Model file for the job. Use its own axes, mm. Face numbers are marked on the shaded views. A direction names the side the tool comes from. Give positions to 0.01 mm unless a question says otherwise; leave off trailing zeros. Order: outer loops, then holes, each group sorted by start corner. A loop starts at its lowest first (then second) coordinate and runs counter-clockwise, first axis right, second up. Notation, with made-up numbers: (87.5, 25.25) - (94.5, 25.25) arc R8 ccw to (94.5, 36.25) - close; hole circle Ø9 at (14, 69). An arc over 180 degrees is marked (long way). Use CSV: the item, a comma, the result in double quotes. Start each with the question number.
(1) Band-saw the part on B-B, the plane x = 1. Give the cut face in (y, z).
(2) Band-saw the part on A-A, the plane z = 4. Give the cut face in (x, y).
(3) Probe L1, parallel to X at y = -6, z = 5.25; L2, parallel to X at y = -10, z = 2; L3, parallel to Y at x = 3, z = 5.75. List the from-to ranges inside material, lowest first.
(4) Band-saw the part on D-D, the plane y = -6. Give the cut face in (x, z), then the cut area to 3 significant figures.
(5) Band-saw the part on C-C, the plane z = 0.5. Give the cut face in (x, y).
(6) Drop flat-ended pins along their axis: pin 1 Ø4.5 at (x, y) = (3.5, -4) entering from +Z; pin 2 Ø2 at (x, z) = (29, 5) entering from -Y. Give the stop position or say it passes through.
(7) Tool access for the marked faces 4, 5 and 6: list every direction of +Z, -Z, +X, -X, +Y, -Y with a clear straight run to the whole face (end or side of a thin tool).
(8) Pull direction X, two halves, no side cores. Call the marked faces 1, 2 and 3: +X half, -X half, draft (parallel to the pull), parting line (faces both ways), or undercut.
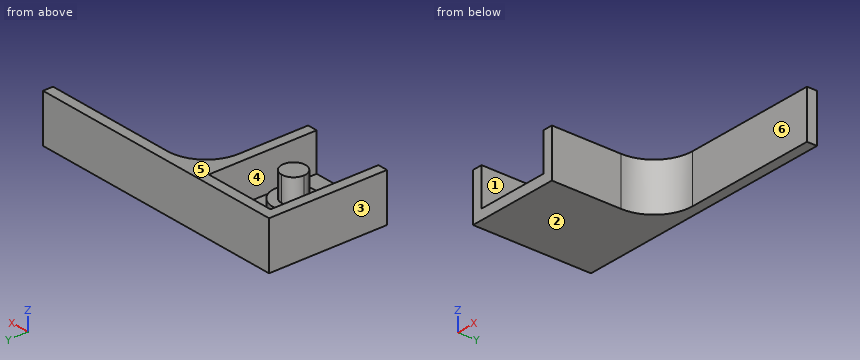
from build123d import *

# Parameters (mm, degrees)
F1_DEPTH = 6.2
F0_W     = 1.3
F0_H     = 14
F2_DEPTH = 3
F3_DEPTH = 1.3
F4_R     = 5


with BuildPart() as f1:
    # F0 (on Top) → F1 (new body)
    with BuildSketch(Plane.XY):
        with BuildLine():
            ThreePointArc((6.25, -7), (5.7960155108, -5.9039844892), (4.7, -5.45))
            Line((4.7, -5.45), (4.7, -7))
            Line((4.7, -7), (3.15, -7))
            ThreePointArc((3.15, -7), (4.7, -8.55), (6.25, -7))
        make_face()
        with BuildLine():
            Line((4.7, -7), (4.7, -5.45))
            ThreePointArc((4.7, -5.45), (3.6039844892, -5.9039844892), (3.15, -7))
            Line((3.15, -7), (4.7, -7))
        make_face()
    extrude(amount=F1_DEPTH)

    # F0 (on Top) → F2 (join)
    with BuildSketch(Plane.XY):
        with BuildLine():
            ThreePointArc((7.4, -7), (6.6091883092, -5.0908116908), (4.7, -4.3))
            Line((4.7, -4.3), (4.7, -5.45))
            ThreePointArc((4.7, -5.45), (5.7960155108, -5.9039844892), (6.25, -7))
            ThreePointArc((6.25, -7), (4.7, -8.55), (3.15, -7))
            Line((3.15, -7), (2, -7))
            ThreePointArc((2, -7), (4.7, -9.7), (7.4, -7))
        make_face()
        with BuildLine():
            Line((4.7, -5.45), (4.7, -4.3))
            ThreePointArc((4.7, -4.3), (2.7908116908, -5.0908116908), (2, -7))
            Line((2, -7), (3.15, -7))
            ThreePointArc((3.15, -7), (3.6039844892, -5.9039844892), (4.7, -5.45))
        make_face()
    extrude(amount=F2_DEPTH)



with BuildPart() as f1b:
    # F0 (on Top) → F1, piece 2 (new body)
    with BuildSketch(Plane.XY):
        Polygon((0, -7), (0, 0), (-1.3, 0), (-1.3, -14), (0, -14), align=None)
        with Locations((10.05, -7)):
            Rectangle(F0_W, F0_H)
        Polygon((-1.3, 0), (0, 0), (4.7, 0), (9.4, 0), (10.7, 0), (33.1, 0), (33.1, 1.3), (-1.3, 1.3), align=None)
    extrude(amount=F1_DEPTH)


with BuildPart() as f1_1:
    add(f1.part)

    add(f1b.part)  # F3 merges F1b
    # F0 (on Top) → F3 (join)
    with BuildSketch(Plane.XY):
        with BuildLine():
            Line((9.4, 0), (4.7, 0))
            Line((4.7, 0), (4.7, -4.3))
            ThreePointArc((4.7, -4.3), (6.6091883092, -5.0908116908), (7.4, -7))
            ThreePointArc((7.4, -7), (4.7, -9.7), (2, -7))
            Line((2, -7), (0, -7))
            Line((0, -7), (0, -14))
            Line((0, -14), (9.4, -14))
            Line((9.4, -14), (9.4, 0))
        make_face()
        with BuildLine():
            Line((4.7, 0), (0, 0))
            Line((0, 0), (0, -7))
            Line((0, -7), (2, -7))
            ThreePointArc((2, -7), (2.7908116908, -5.0908116908), (4.7, -4.3))
            Line((4.7, -4.3), (4.7, 0))
        make_face()
    extrude(amount=F3_DEPTH)

    # F4
    f4_edges = [f1_1.edges().sort_by_distance(p)[0] for p in [
        (10.7, 0, 3.1),
    ]]
    fillet(f4_edges, radius=F4_R)


solid = f1_1.part
Answer block:
1,outline,"(-14, 0) - (1.3, 0) - (1.3, 6.2) - (0, 6.2) - (0, 1.3) - (-14, 1.3) - close"
2,outline,"(-1.3, -14) - (0, -14) - (0, 0) - (9.4, 0) - (9.4, -14) - (10.7, -14) - (10.7, -5) arc R5 cw to (15.7, 0) - (33.1, 0) - (33.1, 1.3) - (-1.3, 1.3) - close; circle Ø3.1 at (4.7, -7)"
3,L1,"x = -1.3 to 0, 3.52 to 5.88, 9.4 to 10.7"
3,L2,"x = -1.3 to 0, 9.4 to 10.7"
3,L3,"y = 0 to 1.3"
4,outline,"(-1.3, 0) - (10.7, 0) - (10.7, 6.2) - (9.4, 6.2) - (9.4, 1.3) - (7.21, 1.3) - (7.21, 3) - (5.88, 3) - (5.88, 6.2) - (3.52, 6.2) - (3.52, 3) - (2.19, 3) - (2.19, 1.3) - (0, 1.3) - (0, 6.2) - (-1.3, 6.2) - close"
4,area,"44.4 mm2"
5,outline,"(-1.3, -14) - (10.7, -14) - (10.7, -5) arc R5 cw to (15.7, 0) - (33.1, 0) - (33.1, 1.3) - (-1.3, 1.3) - close"
6,pin 1,"stops at z = 6.2"
6,pin 2,"stops at y = 0"
7,face 4,"+Z, -Y"
7,face 5,"+Z, +X, -X, +Y, -Y"
7,face 6,"+Z, -Z, +X, -Y"
8,face 1,"undercut"
8,face 2,"draft"
8,face 3,"-X half"
